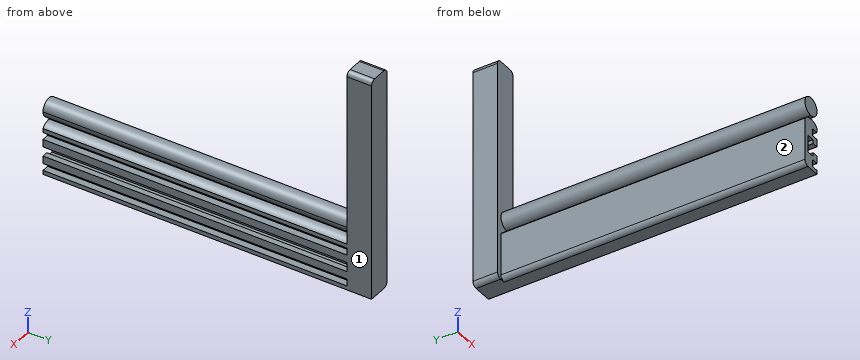
from build123d import *

# Parameters (mm, degrees)
F1_DEPTH = 130
F2_W     = 7.8
F2_H     = 75
F2_H_2   = 20
F3_DEPTH = 10.5
F5_DEPTH = 130
F6_R     = 2
F7_R     = 2


with BuildPart() as f1:
    # F0 (on Front) → F1 (new body)
    with BuildSketch(Plane.XZ):
        Polygon((0, 10), (0, 0), (7.8, 0), (7.8, 1.75), (4.8, 1.75), (4.8, 4.75), (7.8, 4.75), (7.8, 8), (5.3, 8), (5.3, 6.35), (2, 6.35), (2, 10), align=None)
        Polygon((0, 20), (0, 10), (2, 10), (2, 13.65), (5.3, 13.65), (5.3, 12), (7.8, 12), (7.8, 15.25), (4.8, 15.25), (4.8, 18.25), (7.8, 18.25), (7.8, 20), align=None)
    extrude(amount=F1_DEPTH)

    # F2 (on face) → F3 (join)
    with BuildSketch(Plane(origin=(0, 0, 0), x_dir=(-1, 0, 0), z_dir=(0, 1, 0))):
        with Locations((-3.9, 57.5)):
            Rectangle(F2_W, F2_H)
        with Locations((-3.9, 10)):
            Rectangle(F2_W, F2_H_2)
        Polygon((0, 95), (0, 20), (0, 0), (2.2, 0), (2.2, 95), align=None)
    extrude(amount=F3_DEPTH)

    # F4 (on face) → F5 (join, through all)
    with BuildSketch(Plane.XZ):
        with BuildLine():
            Line((3.9, 20), (7.8, 20))
            ThreePointArc((7.8, 20), (6.062812, 21.379122), (3.9, 21.871102))
            Line((3.9, 21.871102), (3.9, 20))
        make_face()
        with BuildLine():
            Line((3.9, 20), (3.9, 21.871102))
            ThreePointArc((3.9, 21.871102), (1.737188, 21.379122), (0, 20))
            Line((0, 20), (3.9, 20))
        make_face()
        with BuildLine():
            ThreePointArc((3.9, 23.371102), (6.657716, 24.513386), (7.8, 27.271102))
            ThreePointArc((7.8, 27.271102), (1.142284, 30.028819), (3.9, 23.371102))
        make_face()
    extrude(amount=F5_DEPTH)

    # F6
    f6_edges = [f1.edges().sort_by_distance(p)[0] for p in [
        (0, -65, 0),
        (7.8, 5.25, 95),
        (-2.2, 5.25, 95),
    ]]
    fillet(f6_edges, radius=F6_R)

    # F7
    f7_edges = [f1.edges().sort_by_distance(p)[0] for p in [
        (-2.2, 5.25, 0),
    ]]
    fillet(f7_edges, radius=F7_R)


solid = f1.part
CAD build for the part. Positions are in the model's coordinates, mm. Face numbers are marked on the shaded views. A direction names the side the tool comes from. Give positions to 0.01 mm unless a question says otherwise; leave off trailing zeros. Loops run counter-clockwise (first coordinate to the right, second up) from the corner with the lowest first, then second, coordinate; pieces in that order, holes last. Notation, with made-up numbers: M 40.5,-13.5 L 86.5,-13.5 A12 cw 86.5,2.5 Z; hole C 46.25,55 d2. An arc over 180 degrees is marked long. One line per question, with ' | ' between items. Start each with the question number.
1. Saw through at B-B on z = 80. Give the cut face in (x, y), plus the area to 3 significant figures.
2. Saw through at A-A on y = -64. Give the cut face in (x, z), plus the area to 3 significant figures.
3. Probe L1, parallel to Z at x = 4.25, y = -85.5; L2, parallel to Z at x = 7.25, y = -70; L3, parallel to Z at x = 5.75, y = -99.5. List the from-to ranges inside material, lowest first. Write a range as from..to.
4. 3-axis set-ups, long thin cutter, end or side, ignore diameter. For the marked faces 1 and 2: which of +Z, -Z, +X, -X, +Y, -Y reach the whole face in a straight line?
5. Flat gauge pins, fed straight in: pin 1 (4.5 mm diameter, centred on x = 3.5, z = 8.5, fed in from -Y); pin 2 (1.6 mm diameter, centred on x = 4, y = -75, fed in from +Z); pin 3 (0.8 mm diameter, centred on x = 6, y = -39, fed in from +Z); pin 4 (1.3 mm diameter, centred on y = -45, z = 7, fed in from -X). Where does each tip first touch, or does it go through?
Result sheet:
1) outline: M -2.2,0 L 7.8,0 L 7.8,10.5 L -2.2,10.5 Z | area: 105 mm^2
2) outline: M 0,2 A2 ccw 2,0 L 7.8,0 L 7.8,1.75 L 4.8,1.75 L 4.8,4.75 L 7.8,4.75 L 7.8,8 L 5.3,8 L 5.3,6.35 L 2,6.35 L 2,13.65 L 5.3,13.65 L 5.3,12 L 7.8,12 L 7.8,15.25 L 4.8,15.25 L 4.8,18.25 L 7.8,18.25 L 7.8,20 A5 ccw 0,20 Z; M 3.9,23.37 A3.9 ccw 7.8,27.27 A3.9 ccw long Z | area: 161 mm^2
3) L1: z = 0..6.35, 13.65..21.86, 23.39..31.16 | L2: z = 0..1.75, 4.75..8, 12..15.25, 18.25..20.58, 25.27..29.27 | L3: z = 0..1.75, 4.75..8, 12..15.25, 18.25..21.52, 23.84..30.7
4) face 1: +Z, -Z, +X, +Y, -Y | face 2: +Z, -Z, -X, -Y
5) pin 1: stops at y = -130 | pin 2: stops at z = 31.17 | pin 3: stops at z = 30.78 | pin 4: stops at x = 0
